Part model, mm, in its own coordinate system. A direction names the side the tool comes from. Round coordinates to 2 decimals unless told otherwise and drop trailing zeros. Order: outer loops, then holes, each group sorted by start corner. A loop starts at its lowest first (then second) coordinate and runs counter-clockwise, first axis right, second up. Notation, with made-up numbers: (42.25, -17.5) - (96.25, -17.5) arc R7 cw to (96.25, -8.5) - close; hole circle Ø3 at (36.5, 66.5). An arc over 180 degrees is marked (long way). Return JSON: item names as keys, results as strings. Group by question number.
Item 1: Tool access for faces 1 (the face through (0.07, 11.11, -2.35)), 2 (the face through (0, -30, -2.072)), 3 (the face through (0, 1, 5)): list every direction of +Z, -Z, +X, -X, +Y, -Y with a clear straight run to the whole face (end or side of a thin tool).
Item 2: Saw through at B-B on x = 0. State how many separate pieces and enclosed holes the cut face has, and give its area (3 significant figures).
Item 3: Saw through at C-C on y = -8. List the corners of the cut face in (x, z).
Item 4: Saw through at A-A on y = -32.5. List the corners of the cut face in (x, z).
Item 5: Probe probe 1 along Z at (x, y) = (-3.5, -22); probe 2 along X at (y, z) = (-5.5, -1); probe 3 along Z at (x, y) = (4, -33.5). List the from-to ranges inside material, lowest first.
Item 6: Saw through at D-D on x = -8. List the corners of the cut face in (y, z), and give its area (3 significant figures).
Item 7: Drop flat-ended pins along their axis: pin 1 (5 mm diameter, centred on x = -12, z = -3.5, fed in from +Y); pin 2 (3 mm diameter, centred on y = 0, z = 2.5, fed in from +X); pin 3 (6 mm diameter, centred on y = -13, z = -0.5, fed in from +X); pin 4 (3.5 mm diameter, centred on x = 0, y = -36.53, fed in from -Z). Give the stop position or say it passes through.
Item 8: Two-plate mould, pull along Z, no slides. Class faces 4 (the face through (-11.465, 8.746, -3.153)), 5 (the face through (9, 7, 1)), 6 (the face through (0.07, 13.515, -1.056)), 7 (the face through (0, -30, 4)): released by +Z, released by -Z, zero draft, split by the parting line, or undercut.
```python
from build123d import *

# Parameters (mm, degrees)
EXTRUDE_1_DEPTH     = 3
EXTRUDE_2_DEPTH     = 14
EXTRUDE_3_DEPTH     = 60
SKETCH_4_R          = 2.3
CUT_EXTRUDE_1_DEPTH = 60
SKETCH_6_W          = 4
SKETCH_6_H          = 10.529479437
CUT_EXTRUDE_2_DEPTH = 60
CUT_EXTRUDE_4_DEPTH = 60


with BuildPart() as part:
    # 草图1 → 凸台-拉伸1 (new body)
    with BuildSketch(Plane(origin=(0, 0, 0), x_dir=(1, 0, 0), z_dir=(0, 1, 0))):
        with BuildLine():
            Line((-12.5, 5), (12.5, 5))
            ThreePointArc((12.5, 5), (17.5, 0), (12.5, -5))
            Line((12.5, -5), (-12.5, -5))
            ThreePointArc((-12.5, -5), (-17.5, 0), (-12.5, 5))
        make_face()
    extrude(amount=EXTRUDE_1_DEPTH)

    # 草图2 → 凸台-拉伸2 (add, symmetric)
    with BuildSketch(Plane(origin=(0, 0, 0), x_dir=(0, 0, -1), z_dir=(1, 0, 0))):
        with BuildLine():
            Line((-5, 3), (-3.508412685, 10.112107418))
            ThreePointArc((-3.508412685, 10.112107418), (1.143689593, 13.506528918), (5, 9.229494551))
            Line((5, 9.229494551), (5, 3))
            Line((5, 3), (-5, 3))
        make_face()
        Polygon((2.88904253, 7.347609244), (3.424289305, 10.184305249), (1.235261889, 12.066190555), (-1.489012301, 11.111379858), (-2.024259076, 8.274683853), (0.164768339, 6.392798546), align=None, mode=Mode.SUBTRACT)
    extrude(amount=EXTRUDE_2_DEPTH, both=True)

    # 草图3 → 凸台-拉伸3 (add)
    with BuildSketch(Plane.XZ):
        with BuildLine():
            Line((-2.5, 4), (2.5, 4))
            ThreePointArc((2.5, 4), (6.5, 0), (2.5, -4))
            Line((2.5, -4), (-2.5, -4))
            ThreePointArc((-2.5, -4), (-6.5, 0), (-2.5, 4))
        make_face()
        with BuildLine():
            Line((-2.705614888, 2.07197125), (2.705614888, 2.07197125))
            ThreePointArc((2.705614888, 2.07197125), (4.777586138, 0), (2.705614888, -2.07197125))
            Line((2.705614888, -2.07197125), (-2.705614888, -2.07197125))
            ThreePointArc((-2.705614888, -2.07197125), (-4.777586138, 0), (-2.705614888, 2.07197125))
        make_face(mode=Mode.SUBTRACT)
    extrude(amount=EXTRUDE_3_DEPTH)

    # 草图4 → 切除-拉伸1 (cut)
    with BuildSketch(Plane.XY.offset(4)):
        with Locations((0, -6.528023855)):
            Circle(SKETCH_4_R)
        with Locations((0, -16.528023855)):
            Circle(SKETCH_4_R)
        with Locations((0, -26.528023855)):
            Circle(SKETCH_4_R)
        with Locations((0, -36.528023855)):
            Circle(SKETCH_4_R)
        with Locations((0, -46.528023855)):
            Circle(SKETCH_4_R)
        with Locations((0, -56.528023855)):
            Circle(SKETCH_4_R)
    extrude(amount=-CUT_EXTRUDE_1_DEPTH, mode=Mode.SUBTRACT)

    # 草图6 → 切除-拉伸2 (cut)
    with BuildSketch(Plane(origin=(0, 0, -5), x_dir=(-1, 0, 0), z_dir=(0, 0, -1))):
        with Locations((-7, 8.264739718)):
            Rectangle(SKETCH_6_W, SKETCH_6_H)
        with Locations((7, 8.264739718)):
            Rectangle(SKETCH_6_W, SKETCH_6_H)
    extrude(amount=-CUT_EXTRUDE_2_DEPTH, mode=Mode.SUBTRACT)

    # 草图7 → 切除-拉伸4 (cut)
    with BuildSketch(Plane.XZ):
        with BuildLine():
            Line((-21.020097189, 8.097906294), (21.020097189, 8.097906294))
            ThreePointArc((21.020097189, 8.097906294), (29.118003483, 0), (21.020097189, -8.097906294))
            Line((21.020097189, -8.097906294), (-21.020097189, -8.097906294))
            ThreePointArc((-21.020097189, -8.097906294), (-29.118003483, 0), (-21.020097189, 8.097906294))
        make_face()
        with BuildLine():
            Line((-12.5, -5), (12.5, -5))
            ThreePointArc((12.5, -5), (17.5, 0), (12.5, 5))
            Line((12.5, 5), (-12.5, 5))
            ThreePointArc((-12.5, 5), (-17.5, 0), (-12.5, -5))
        make_face(mode=Mode.SUBTRACT)
    extrude(amount=-CUT_EXTRUDE_4_DEPTH, mode=Mode.SUBTRACT)


solid = part.part
```
Filled in:
{
 "1": {"face 1": "+X, -X", "face 2": "-Y", "face 3": "+Z, +X, -X, +Y, -Y"},
 "2": {"separate pieces": "13", "enclosed holes": "1", "area": "221 mm^2"},
 "3": {"outline": "(-2.71, -2.07) arc R2.07 cw to (-2.71, 2.07) - (-1.77, 2.07) - (-1.77, 4) - (-2.5, 4) arc R4 ccw to (-2.5, -4) - (-1.77, -4) - (-1.77, -2.07) - close; (1.77, -4) - (2.5, -4) arc R4 ccw to (2.5, 4) - (1.77, 4) - (1.77, 2.07) - (2.71, 2.07) arc R2.07 cw to (2.71, -2.07) - (1.77, -2.07) - close"},
 "4": {"outline": "(-2.5, -4) - (2.5, -4) arc R4 ccw to (2.5, 4) - (-2.5, 4) arc R4 ccw to start; hole (-2.71, -2.07) - (2.71, -2.07) arc R2.07 ccw to (2.71, 2.07) - (-2.71, 2.07) arc R2.07 ccw to start"},
 "5": {"probe 1": "z = -3.87 to -1.91, 1.91 to 3.87", "probe 2": "x = -6.37 to -4.52, 4.52 to 6.37", "probe 3": "z = -3.71 to -1.62, 1.62 to 3.71"},
 "6": {"outline": "(0, -5) - (3, -5) - (3, 5) - (0, 5) - close", "area": "30.0 mm^2"},
 "7": {"pin 1": "stops at y = 13.52", "pin 2": "stops at x = 17.4", "pin 3": "stops at x = 6.5", "pin 4": "passes through"},
 "8": {"face 4": "undercut", "face 5": "zero draft", "face 6": "split by the parting line", "face 7": "released by +Z"}
}
